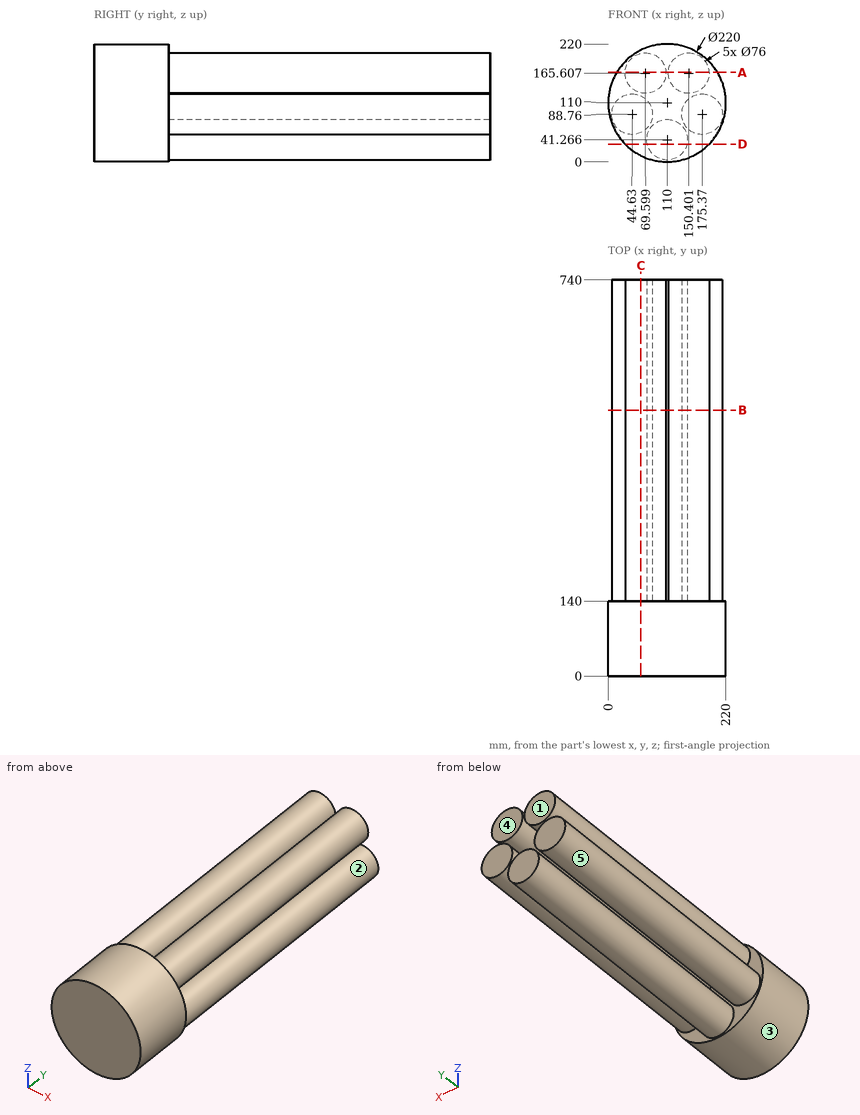
For this review, use the dimensioned drawing (mm, ordinates from the lowest corner) and the shaded views. A direction names the side the tool comes from. Give positions to 0.01 mm unless a question says otherwise; leave off trailing zeros. Write each loop counter-clockwise with the first axis right and the second up, starting at its lowest first coordinate (ties: lowest second). Pieces come first, ordered by that corner, then holes.
(1) For P1, Ø1.5, axis at x = 145.5, y = 509.5, coming from the +Z side; P2, Ø8, axis at y = 548.5, z = 35.5, coming from the +X side; P3, Ø1, axis at y = 246.5, z = 84, coming from the -X side, all flat-tipped, find the tip position at first contact; note any pin that passes through.
(2) Consider section A-A, the plane z = 167. Give the boundary of the cut face in (x, y) (1 decimal).
(3) To check wall thickness, follow L1, parallel to X at y = 238, z = 89.5; L2, parallel to X at y = 182, z = 165.5; L3, parallel to Y at x = 97, z = 205.5. State the ranges of each line that lie inside material, in increasing order.
(4) Consider section D-D, the plane z = 33. Give the boundary of the cut face in (x, y).
(5) Consider section B-B, the plane y = 496.5. Give the boundary of the cut face in (x, z) (1 decimal), and give its area (3 significant figures).
(6) The part is to be moulded in two halves that separate along X. For the marked faces 3, 4 and 5, say which applies: released by +X, released by -X, zero draft, split by the parting line, or undercut.
(7) Tool access review of the marked faces 1 and 2: name each direction out of +Z, -Z, +X, -X, +Y, -Y from which nothing blocks a thin tool from reaching the whole face with its end or side.
(8) Consider section C-C, the plane x = 61. Give the boundary of the cut face in (y, z).
Returned:
1. P1: stops at z = 203.38
1. P2: stops at x = 147.96
1. P3: stops at x = 6.87
2. outline: (15.9, 0) - (204.1, 0) - (204.1, 140) - (188.4, 140) - (188.4, 740) - (112.4, 740) - (112.4, 140) - (107.6, 140) - (107.6, 740) - (31.6, 740) - (31.6, 140) - (15.9, 140) - close
3. L1: x = 6.64 to 82.62, 137.38 to 213.36
3. L2: x = 31.6 to 107.6, 112.4 to 188.4
3. L3: y = 0 to 140
4. outline: (31.44, 0) - (188.56, 0) - (188.56, 140) - (147.09, 140) - (147.09, 740) - (72.91, 740) - (72.91, 140) - (31.44, 140) - close
5. outline: circle Ø76 at (44.6, 88.8); circle Ø76 at (69.6, 165.6); circle Ø76 at (110, 41.3); circle Ø76 at (150.4, 165.6); circle Ø76 at (175.4, 88.8)
5. area: 22,700 mm2
6. face 3: split by the parting line
6. face 4: zero draft
6. face 5: undercut
7. face 1: +Z, -Z, +X, -X, +Y
7. face 2: +Y
8. outline: (0, 11.52) - (140, 11.52) - (140, 54.47) - (740, 54.47) - (740, 123.05) - (140, 123.05) - (140, 128.59) - (740, 128.59) - (740, 202.62) - (140, 202.62) - (140, 208.48) - (0, 208.48) - close
